```python
from build123d import *

# Parameters (mm, degrees)
CROQUIS1_R              = 87.5
SALIENTE_EXTRUIR1_DEPTH = 3.75
CROQUIS2_R              = 8.3
CORTAR_EXTRUIR1_DEPTH   = 1.5
CROQUIS3_R              = 5.25
CORTAR_EXTRUIR2_DEPTH   = 4.75
MATRIZC1_COUNT          = 8


with BuildPart() as part:
    # Croquis1 → Saliente-Extruir1 (new body)
    with BuildSketch(Plane.XY):
        Circle(CROQUIS1_R)
        with BuildLine():
            ThreePointArc((-38.757376395, -22.5), (-31.688990399, -31.688990399), (-22.5, -38.757376395))
            ThreePointArc((-22.5, -38.757376395), (-15.606593782, -38.639265866), (-12.5, -32.484424319))
            ThreePointArc((-12.5, -32.484424319), (-10.144121841, -26.518786087), (-4, -24.677925359))
            ThreePointArc((-4, -24.677925359), (0, -25), (4, -24.677925359))
            ThreePointArc((4, -24.677925359), (10.144121841, -26.518786087), (12.5, -32.484424319))
            ThreePointArc((12.5, -32.484424319), (15.606593782, -38.639265866), (22.5, -38.757376395))
            ThreePointArc((22.5, -38.757376395), (31.688990399, -31.688990399), (38.757376395, -22.5))
            ThreePointArc((38.757376395, -22.5), (38.639265866, -15.606593782), (32.484424319, -12.5))
            ThreePointArc((32.484424319, -12.5), (26.518786087, -10.144121841), (24.677925359, -4))
            ThreePointArc((24.677925359, -4), (25, 0), (24.677925359, 4))
            ThreePointArc((24.677925359, 4), (26.518786087, 10.144121841), (32.484424319, 12.5))
            ThreePointArc((32.484424319, 12.5), (38.639265866, 15.606593782), (38.757376395, 22.5))
            ThreePointArc((38.757376395, 22.5), (31.688990399, 31.688990399), (22.5, 38.757376395))
            ThreePointArc((22.5, 38.757376395), (15.606593782, 38.639265866), (12.5, 32.484424319))
            ThreePointArc((12.5, 32.484424319), (10.144121841, 26.518786087), (4, 24.677925359))
            ThreePointArc((4, 24.677925359), (0, 25), (-4, 24.677925359))
            ThreePointArc((-4, 24.677925359), (-10.144121841, 26.518786087), (-12.5, 32.484424319))
            ThreePointArc((-12.5, 32.484424319), (-15.606593782, 38.639265866), (-22.5, 38.757376395))
            ThreePointArc((-22.5, 38.757376395), (-31.688990399, 31.688990399), (-38.757376395, 22.5))
            ThreePointArc((-38.757376395, 22.5), (-38.639265866, 15.606593782), (-32.484424319, 12.5))
            ThreePointArc((-32.484424319, 12.5), (-26.518786087, 10.144121841), (-24.677925359, 4))
            ThreePointArc((-24.677925359, 4), (-25, 0), (-24.677925359, -4))
            ThreePointArc((-24.677925359, -4), (-26.518786087, -10.144121841), (-32.484424319, -12.5))
            ThreePointArc((-32.484424319, -12.5), (-38.639265866, -15.606593782), (-38.757376395, -22.5))
        make_face(mode=Mode.SUBTRACT)
    extrude(amount=SALIENTE_EXTRUIR1_DEPTH)

    # Croquis2 → Cortar-Extruir1 (cut)
    with BuildSketch(Plane.XY.offset(3.75)):
        with Locations((-36.515, 0)):
            Circle(CROQUIS2_R)
        with Locations((0, 36.515)):
            Circle(CROQUIS2_R)
        with Locations((36.515, 0)):
            Circle(CROQUIS2_R)
        with Locations((0, -36.515)):
            Circle(CROQUIS2_R)
    extrude(amount=-CORTAR_EXTRUIR1_DEPTH, mode=Mode.SUBTRACT)

    # Croquis3 → Cortar-Extruir2 (cut, through all)
    with BuildSketch(Plane.XY.offset(3.75)):
        with Locations((0, 36.515)):
            Circle(CROQUIS3_R)
    cortar_extruir2 = extrude(amount=-CORTAR_EXTRUIR2_DEPTH, mode=Mode.SUBTRACT)

    # MatrizC1: Cortar-Extruir2 ×8 about axis
    matrizc1_axis = Axis((0, 0, 3.75), (0, 0, 1))
    for i in range(1, MATRIZC1_COUNT):
        add(cortar_extruir2.rotate(matrizc1_axis, i * 360 / MATRIZC1_COUNT), mode=Mode.SUBTRACT)


solid = part.part
```
Source: CAD feature listing. Evaluate the final solid. Frame: model axes, mm. A direction names the side the tool comes from. Round coordinates to 2 decimals unless told otherwise and drop trailing zeros. Loops run counter-clockwise (first coordinate to the right, second up) from the corner with the lowest first, then second, coordinate; pieces in that order, holes last.
1. Section query C-C on z = 1.15. Give the number of separate pieces and of enclosed holes in the cut face, and give its area (3 significant figures).
2. Ray query, L1, parallel to Y at x = 0, z = 3.1 (3 decimals); L2, parallel to X at y = 0.5, z = 3.35 (3 decimals); L3, parallel to Y at x = 0, z = 0.7 (3 decimals). Return the intervals inside material, ascending.
3. Section query D-D on x = 58. Output: boundary loops of the cut face in (y, z), and give its area (3 significant figures).
4. Access query for faces 1 (the cylindrical face through (31.804, 31.574, 1.849)), 2 (the flat face through (0, 31, 2.25)). Directions: +Z, -Z, +X, -X, +Y, -Y. A direction counts if a zero-diameter tool reaches every point of the face in a straight line with its end or side. Return the directions, or none.
5. Section query A-A on y = 0. Output: boundary loops of the cut face in (x, z) (3 decimals).
6. Contact query for flat-ended pins moving along their axis: pin 1 (13.5 mm diameter, centred on x = -0.5, y = -37, fed in from +Z); pin 2 (13.5 mm diameter, centred on x = 34, y = 4, fed in from +Z); pin 3 (1 mm diameter, centred on y = 57.5, z = 2, fed in from -X). Output: stop coordinate, or through.
Answers below:
1. separate pieces: 1
1. enclosed holes: 5
1. area: 19,500 mm2
2. L1: y = -87.5 to -44.815, -28.215 to -25, 25 to 28.215, 44.815 to 87.5
2. L2: x = -87.499 to -44.8, -28.23 to -24.995, 24.995 to 28.23, 44.8 to 87.499
2. L3: y = -87.5 to -41.765, -31.265 to -25, 25 to 31.265, 41.765 to 87.5
3. outline: (-65.52, 0) - (65.52, 0) - (65.52, 3.75) - (-65.52, 3.75) - close
3. area: 491 mm2
4. face 1: +Z, -Z
4. face 2: +Z
5. outline: (-87.5, 0) - (-41.765, 0) - (-41.765, 2.25) - (-44.815, 2.25) - (-44.815, 3.75) - (-87.5, 3.75) - close; (-31.265, 0) - (-25, 0) - (-25, 3.75) - (-28.215, 3.75) - (-28.215, 2.25) - (-31.265, 2.25) - close; (25, 0) - (31.265, 0) - (31.265, 2.25) - (28.215, 2.25) - (28.215, 3.75) - (25, 3.75) - close; (41.765, 0) - (87.5, 0) - (87.5, 3.75) - (44.815, 3.75) - (44.815, 2.25) - (41.765, 2.25) - close
6. pin 1: stops at z = 2.25
6. pin 2: stops at z = 3.75
6. pin 3: stops at x = -66.39
